Can you work these out from the model? Positions are in its coordinate system, mm. Face numbers are marked on the shaded views. A direction names the side the tool comes from. Round coordinates to 2 decimals unless told otherwise and drop trailing zeros. Loops run counter-clockwise (first coordinate to the right, second up) from the corner with the lowest first, then second, coordinate; pieces in that order, holes last. Notation, with made-up numbers: (16, 85.5) - (55, 85.5) arc R4 ccw to (55, 91.5) - close; hole circle Ø8 at (1.5, 39.25). An arc over 180 degrees is marked (long way). Answer as CSV lines item,"result".
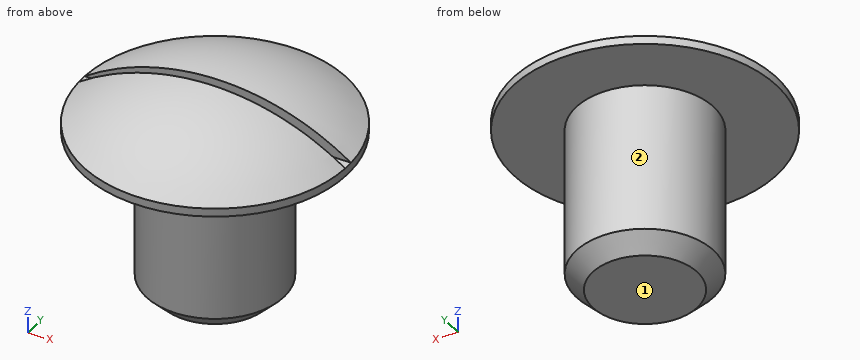
```python
from build123d import *

# Parameters (mm, degrees)
SKETCH4_R               = 5.30225
BOSS_EXTRUDE3_DEPTH     = 12.7
CUT_EXTRUDE1_DEPTH      = 0.381
CUT_EXTRUDE1_DEPTH_BACK = 0.381
SKETCH6_W               = 20.32
SKETCH6_H               = 5.08
CHAMFER1_SIZE           = 1.27


with BuildPart() as part:
    # Sketch4 → Boss-Extrude3 (new body)
    with BuildSketch(Plane.XY):
        Circle(SKETCH4_R)
    extrude(amount=-BOSS_EXTRUDE3_DEPTH)

    # Sketch5 → Revolve2 (revolve)
    with BuildSketch(Plane(origin=(0, 0, 0), x_dir=(1, 0, 0), z_dir=(0, 1, 0)), mode=Mode.PRIVATE) as revolve2_sk:
        with BuildLine():
            Line((-10.16, 0), (-10.16, -0.635))
            ThreePointArc((-10.16, -0.635), (-5.32226984, -2.997763488), (0, -3.81))
            Line((0, -3.81), (0, 0))
            Line((0, 0), (-10.16, 0))
        make_face()
    revolve(revolve2_sk.sketch.rotate(Axis((0, 0, 0), (0, 0, 1)), 180), axis=Axis((0, 0, 0), (0, 0, 1)))

    # Sketch6 → Cut-Extrude1 (cut, two sides: drawn at the far end of the back side and taken through both)
    with BuildSketch(Plane(origin=(0, 0, 0), x_dir=(1, 0, 0), z_dir=(0, 1, 0)).offset(-CUT_EXTRUDE1_DEPTH_BACK)):
        with Locations((0, -3.175)):
            Rectangle(SKETCH6_W, SKETCH6_H)
    extrude(amount=CUT_EXTRUDE1_DEPTH + CUT_EXTRUDE1_DEPTH_BACK, mode=Mode.SUBTRACT)

    # Chamfer1
    chamfer1_edges = [part.edges().sort_by_distance(p)[0] for p in [
        (-5.30225, 0, -12.7),
    ]]
    chamfer(chamfer1_edges, length=CHAMFER1_SIZE)


solid = part.part
```
Q1. Imagine slicing it at D-D (z = -0.75). Write out the boundary of the cut face in (x, y).
Checks:
outline,"circle Ø10.6 at (0, 0)"
Q2. Imagine slicing it at C-C (z = 2.5). Write out the boundary of the cut face in (x, y).
Checks:
outline,"(-6.7, -0.38) arc R6.71 ccw to (6.7, -0.38) - close; (-6.7, 0.38) - (6.7, 0.38) arc R6.71 ccw to start"
Q3. On a 3-axis mill with a long thin cutter (end or side, diameter ignored), from which of +Z, -Z, +X, -X, +Y, -Y can I reach the whole of each face in a straight line? I mean the marked faces 1 and 2. Say none if no direction works.
Checks:
face 1,"-Z, +X, -X, +Y, -Y"
face 2,"-Z"
Q4. Imagine slicing it at A-A (y = 0). Write out the boundary of the cut face in (x, z) (3 decimals).
Checks:
outline,"(-10.16, 0) - (-5.302, 0) - (-5.302, -11.43) - (-4.032, -12.7) - (4.032, -12.7) - (5.302, -11.43) - (5.302, 0) - (10.16, 0) - (10.16, 0.635) - (-10.16, 0.635) - close"
Q5. If I drill on line 1 along Y through (x, z) = (0, -6.5); line 2 along Y through (x, z) = (3, 0.75); line 3 along X through (y, z) = (4, -6), over which ranges is the centre line in solid material (lowest first)? Write a range as [from, to].
Checks:
line 1,"[-5.3, 5.3]"
line 2,"[-9.53, -0.38], [0.38, 9.53]"
line 3,"[-3.48, 3.48]"
Q6. I'm going to push flat-ended pins straight in: pin 1 Ø5 at (y, z) = (-0.5, -10) entering from +X; pin 2 Ø8 at (y, z) = (-6, -8) entering from -X; pin 3 Ø0.6 at (x, y) = (2.5, 0) entering from +Z (3 decimals). Where does each tip first touch, or does it pass through?
Checks:
pin 1,"x = 5.3"
pin 2,"x = -4.91"
pin 3,"z = 0.635"
Q7. Imagine slicing it at B-B (x = 0). Write out the boundary of the cut face in (y, z) (1 decimal).
Checks:
outline,"(-10.2, 0) - (-5.3, 0) - (-5.3, -11.4) - (-4, -12.7) - (4, -12.7) - (5.3, -11.4) - (5.3, 0) - (10.2, 0) - (10.2, 0.6) arc R17.8 ccw to (0.4, 3.8) - (0.4, 0.6) - (-0.4, 0.6) - (-0.4, 3.8) arc R17.8 ccw to (-10.2, 0.6) - close"
